Read the model definition and answer for the solid it produces. Units are mm, in the model's axes. Give positions to 0.01 mm unless a question says otherwise; leave off trailing zeros. Loops run counter-clockwise (first coordinate to the right, second up) from the corner with the lowest first, then second, coordinate; pieces in that order, holes last. Notation, with made-up numbers: (87, -36.75) - (141, -36.75) arc R26 cw to (141, -5.75) - close; hole circle Ø5 at (-33.75, 76.25). An arc over 180 degrees is marked (long way). Write each question's results on one line, items separated by ' | '. Start each with the question number.
Q1. The part is cut by section B-B, the plane z = 7. Write down the section's boundary in (x, y) (3 decimals), plus the area to 3 significant figures.
Q2. Given pin 1 (0.8 mm diameter, centred on y = -1, z = 0.5, fed in from -X); pin 2 (1.5 mm diameter, centred on x = 0, y = 0.5, fed in from +Z); pin 3 (1.1 mm diameter, centred on x = -1, z = 0.5, fed in from +Y); pin 4 (0.5 mm diameter, centred on x = 1, z = 0.5, fed in from +Y), each flat-ended and moving along its own axis, determine where each tip first touches the part or whether it passes through.
Q3. Find the intervals of material crossed by line 1 (Y direction, x = -0.25, z = 3); line 2 (Z direction, x = 0, y = -0.1); line 3 (X direction, y = 0.1, z = 0.75), in increasing order. Write a range as from..to.
Q4. The part is cut by section A-A, the plane z = 5. Write down the section's boundary in (x, y).
```python
from build123d import *

# Parameters (mm, degrees)
F0_R     = 2
F1_DEPTH = 1
F2_START = 1
F0_W     = 0.5
F0_H     = 0.5
F2_DEPTH = 0.5
F3_START = 1.5
F3_DEPTH = 8
F4_SIZE2 = 3
F4_SIZE  = 0.75
F6_R     = 0.25


# Not quite as in the source:
# - a fillet or chamfer that OpenCascade refuses, or shapes differently, is made with other operations: its cross-section is extruded or revolved along the edge and cut away or added


with BuildPart() as f1:
    # F0 (on Top) → F1 (new body)
    with BuildSketch(Plane.XY):
        Circle(F0_R)
        with BuildLine():
            ThreePointArc((0.25, 0.9682458366), (0.7071067812, 0.7071067812), (0.9682458366, 0.25))
            Line((0.9682458366, 0.25), (1.25, 0.25))
            Line((1.25, 0.25), (1.25, -0.25))
            Line((1.25, -0.25), (0.9682458366, -0.25))
            ThreePointArc((0.9682458366, -0.25), (0.7071067812, -0.7071067812), (0.25, -0.9682458366))
            Line((0.25, -0.9682458366), (0.25, -1.25))
            Line((0.25, -1.25), (-0.25, -1.25))
            Line((-0.25, -1.25), (-0.25, -0.9682458366))
            ThreePointArc((-0.25, -0.9682458366), (-0.7071067812, -0.7071067812), (-0.9682458366, -0.25))
            Line((-0.9682458366, -0.25), (-1.25, -0.25))
            Line((-1.25, -0.25), (-1.25, 0.25))
            Line((-1.25, 0.25), (-0.9682458366, 0.25))
            ThreePointArc((-0.9682458366, 0.25), (-0.7071067812, 0.7071067812), (-0.25, 0.9682458366))
            Line((-0.25, 0.9682458366), (-0.25, 1.25))
            Line((-0.25, 1.25), (0.25, 1.25))
            Line((0.25, 1.25), (0.25, 0.9682458366))
        make_face(mode=Mode.SUBTRACT)
        with BuildLine():
            Line((-0.25, 0.25), (-0.25, 0.9682458366))
            ThreePointArc((-0.25, 0.9682458366), (-0.7071067812, 0.7071067812), (-0.9682458366, 0.25))
            Line((-0.9682458366, 0.25), (-0.25, 0.25))
        make_face()
        with BuildLine():
            ThreePointArc((-0.9682458366, -0.25), (-0.7071067812, -0.7071067812), (-0.25, -0.9682458366))
            Line((-0.25, -0.9682458366), (-0.25, -0.25))
            Line((-0.25, -0.25), (-0.9682458366, -0.25))
        make_face()
        with BuildLine():
            ThreePointArc((0.25, -0.9682458366), (0.7071067812, -0.7071067812), (0.9682458366, -0.25))
            Line((0.9682458366, -0.25), (0.25, -0.25))
            Line((0.25, -0.25), (0.25, -0.9682458366))
        make_face()
        with BuildLine():
            Line((0.25, 0.25), (0.9682458366, 0.25))
            ThreePointArc((0.9682458366, 0.25), (0.7071067812, 0.7071067812), (0.25, 0.9682458366))
            Line((0.25, 0.9682458366), (0.25, 0.25))
        make_face()
    extrude(amount=F1_DEPTH)

    # F0 (on Top) → F2 (join)
    with BuildSketch(Plane.XY.offset(F2_START)):
        Circle(F0_R)
        with BuildLine():
            ThreePointArc((0.25, 0.9682458366), (0.7071067812, 0.7071067812), (0.9682458366, 0.25))
            Line((0.9682458366, 0.25), (1.25, 0.25))
            Line((1.25, 0.25), (1.25, -0.25))
            Line((1.25, -0.25), (0.9682458366, -0.25))
            ThreePointArc((0.9682458366, -0.25), (0.7071067812, -0.7071067812), (0.25, -0.9682458366))
            Line((0.25, -0.9682458366), (0.25, -1.25))
            Line((0.25, -1.25), (-0.25, -1.25))
            Line((-0.25, -1.25), (-0.25, -0.9682458366))
            ThreePointArc((-0.25, -0.9682458366), (-0.7071067812, -0.7071067812), (-0.9682458366, -0.25))
            Line((-0.9682458366, -0.25), (-1.25, -0.25))
            Line((-1.25, -0.25), (-1.25, 0.25))
            Line((-1.25, 0.25), (-0.9682458366, 0.25))
            ThreePointArc((-0.9682458366, 0.25), (-0.7071067812, 0.7071067812), (-0.25, 0.9682458366))
            Line((-0.25, 0.9682458366), (-0.25, 1.25))
            Line((-0.25, 1.25), (0.25, 1.25))
            Line((0.25, 1.25), (0.25, 0.9682458366))
        make_face(mode=Mode.SUBTRACT)
        with BuildLine():
            Line((0.25, 0.25), (0.25, 0.9682458366))
            ThreePointArc((0.25, 0.9682458366), (0, 1), (-0.25, 0.9682458366))
            Line((-0.25, 0.9682458366), (-0.25, 0.25))
            Line((-0.25, 0.25), (0.25, 0.25))
        make_face()
        with BuildLine():
            ThreePointArc((-0.25, -0.9682458366), (0, -1), (0.25, -0.9682458366))
            Line((0.25, -0.9682458366), (0.25, -0.25))
            Line((0.25, -0.25), (-0.25, -0.25))
            Line((-0.25, -0.25), (-0.25, -0.9682458366))
        make_face()
        with BuildLine():
            ThreePointArc((0.9682458366, -0.25), (0.9920296963, -0.1260042925), (1, 0))
            ThreePointArc((1, 0), (0.9920296963, 0.1260042925), (0.9682458366, 0.25))
            Line((0.9682458366, 0.25), (0.25, 0.25))
            Line((0.25, 0.25), (0.25, -0.25))
            Line((0.25, -0.25), (0.9682458366, -0.25))
        make_face()
        with BuildLine():
            Line((-0.25, -0.25), (-0.25, 0.25))
            Line((-0.25, 0.25), (-0.9682458366, 0.25))
            ThreePointArc((-0.9682458366, 0.25), (-1, 0), (-0.9682458366, -0.25))
            Line((-0.9682458366, -0.25), (-0.25, -0.25))
        make_face()
        with BuildLine():
            ThreePointArc((-0.9682458366, -0.25), (-0.7071067812, -0.7071067812), (-0.25, -0.9682458366))
            Line((-0.25, -0.9682458366), (-0.25, -0.25))
            Line((-0.25, -0.25), (-0.9682458366, -0.25))
        make_face()
        with BuildLine():
            ThreePointArc((0.25, -0.9682458366), (0.7071067812, -0.7071067812), (0.9682458366, -0.25))
            Line((0.9682458366, -0.25), (0.25, -0.25))
            Line((0.25, -0.25), (0.25, -0.9682458366))
        make_face()
        with BuildLine():
            Line((0.25, 0.25), (0.9682458366, 0.25))
            ThreePointArc((0.9682458366, 0.25), (0.7071067812, 0.7071067812), (0.25, 0.9682458366))
            Line((0.25, 0.9682458366), (0.25, 0.25))
        make_face()
        with BuildLine():
            Line((-0.25, 0.25), (-0.25, 0.9682458366))
            ThreePointArc((-0.25, 0.9682458366), (-0.7071067812, 0.7071067812), (-0.9682458366, 0.25))
            Line((-0.9682458366, 0.25), (-0.25, 0.25))
        make_face()
        Rectangle(F0_W, F0_H)
        with BuildLine():
            ThreePointArc((-0.9682458366, -0.25), (-1, 0), (-0.9682458366, 0.25))
            Line((-0.9682458366, 0.25), (-1.25, 0.25))
            Line((-1.25, 0.25), (-1.25, -0.25))
            Line((-1.25, -0.25), (-0.9682458366, -0.25))
        make_face()
        with BuildLine():
            ThreePointArc((0.9682458366, 0.25), (0.9920296963, 0.1260042925), (1, 0))
            ThreePointArc((1, 0), (0.9920296963, -0.1260042925), (0.9682458366, -0.25))
            Line((0.9682458366, -0.25), (1.25, -0.25))
            Line((1.25, -0.25), (1.25, 0.25))
            Line((1.25, 0.25), (0.9682458366, 0.25))
        make_face()
        with BuildLine():
            ThreePointArc((-0.25, 0.9682458366), (0, 1), (0.25, 0.9682458366))
            Line((0.25, 0.9682458366), (0.25, 1.25))
            Line((0.25, 1.25), (-0.25, 1.25))
            Line((-0.25, 1.25), (-0.25, 0.9682458366))
        make_face()
        with BuildLine():
            Line((0.25, -1.25), (0.25, -0.9682458366))
            ThreePointArc((0.25, -0.9682458366), (0, -1), (-0.25, -0.9682458366))
            Line((-0.25, -0.9682458366), (-0.25, -1.25))
            Line((-0.25, -1.25), (0.25, -1.25))
        make_face()
    extrude(amount=F2_DEPTH)

    # F0 (on Top) → F3 (join)
    with BuildSketch(Plane.XY.offset(F3_START)):
        with BuildLine():
            ThreePointArc((-0.9682458366, -0.25), (-0.7071067812, -0.7071067812), (-0.25, -0.9682458366))
            Line((-0.25, -0.9682458366), (-0.25, -0.25))
            Line((-0.25, -0.25), (-0.9682458366, -0.25))
        make_face()
        with BuildLine():
            Line((-0.25, -0.25), (-0.25, 0.25))
            Line((-0.25, 0.25), (-0.9682458366, 0.25))
            ThreePointArc((-0.9682458366, 0.25), (-1, 0), (-0.9682458366, -0.25))
            Line((-0.9682458366, -0.25), (-0.25, -0.25))
        make_face()
        with BuildLine():
            Line((-0.25, 0.25), (-0.25, 0.9682458366))
            ThreePointArc((-0.25, 0.9682458366), (-0.7071067812, 0.7071067812), (-0.9682458366, 0.25))
            Line((-0.9682458366, 0.25), (-0.25, 0.25))
        make_face()
        with BuildLine():
            Line((0.25, 0.25), (0.25, 0.9682458366))
            ThreePointArc((0.25, 0.9682458366), (0, 1), (-0.25, 0.9682458366))
            Line((-0.25, 0.9682458366), (-0.25, 0.25))
            Line((-0.25, 0.25), (0.25, 0.25))
        make_face()
        with BuildLine():
            Line((0.25, 0.25), (0.9682458366, 0.25))
            ThreePointArc((0.9682458366, 0.25), (0.7071067812, 0.7071067812), (0.25, 0.9682458366))
            Line((0.25, 0.9682458366), (0.25, 0.25))
        make_face()
        with BuildLine():
            ThreePointArc((0.9682458366, -0.25), (0.9920296963, -0.1260042925), (1, 0))
            ThreePointArc((1, 0), (0.9920296963, 0.1260042925), (0.9682458366, 0.25))
            Line((0.9682458366, 0.25), (0.25, 0.25))
            Line((0.25, 0.25), (0.25, -0.25))
            Line((0.25, -0.25), (0.9682458366, -0.25))
        make_face()
        with BuildLine():
            ThreePointArc((-0.25, -0.9682458366), (0, -1), (0.25, -0.9682458366))
            Line((0.25, -0.9682458366), (0.25, -0.25))
            Line((0.25, -0.25), (-0.25, -0.25))
            Line((-0.25, -0.25), (-0.25, -0.9682458366))
        make_face()
        with BuildLine():
            ThreePointArc((0.25, -0.9682458366), (0.7071067812, -0.7071067812), (0.9682458366, -0.25))
            Line((0.9682458366, -0.25), (0.25, -0.25))
            Line((0.25, -0.25), (0.25, -0.9682458366))
        make_face()
        Rectangle(F0_W, F0_H)
    extrude(amount=F3_DEPTH)

    # F4
    f4_edges = [f1.edges().sort_by_distance(p)[0] for p in [
        (-0.25, 0.968246, 9.5),
    ]]
    f4_side = f1.faces().sort_by_distance((0, 0, 9.5))[0]
    chamfer(f4_edges, length=F4_SIZE, length2=F4_SIZE2, reference=f4_side)

    # F5: fillet of radius 1 on 1 edges, made by hand

    # F5_s1 → F5_t2 (revolve, cut)
    with BuildSketch(Plane.XZ):
        with BuildLine():
            ThreePointArc((2, 1), (1.7071067812, 0.2928932188), (1, 0))
            Line((1, 0), (2, 0))
            Line((2, 0), (2, 1))
        make_face()
    revolve(axis=Axis((0, 0, 0), (0, 0, 1)), mode=Mode.SUBTRACT)

    # F6
    f6_edges = [f1.edges().sort_by_distance(p)[0] for p in [
        (-2, 0, 1.5),
        (-0.25, 0.968246, 1.5),
    ]]
    fillet(f6_edges, radius=F6_R)


solid = f1.part
```
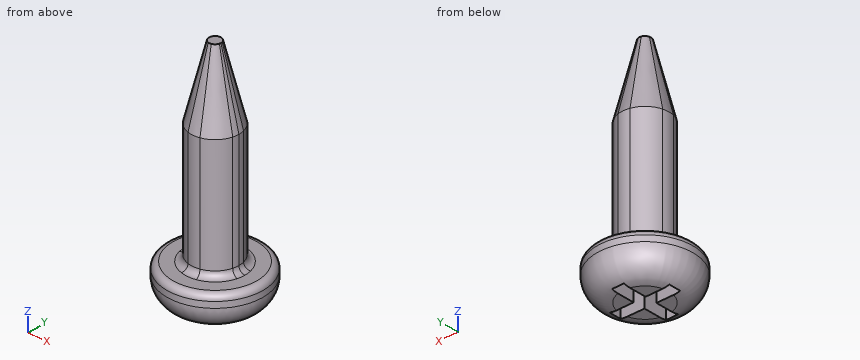
Check sheet entries:
1) outline: circle Ø1.75 at (0, 0) | area: 2.41 mm^2
2) pin 1: stops at x = -1.84 | pin 2: stops at z = 9.5 | pin 3: stops at y = 1.91 | pin 4: stops at y = 1.76
3) line 1: y = -0.97..0.97 | line 2: z = 1..9.5 | line 3: x = -1.97..-1.25, 1.25..1.97
4) outline: circle Ø2 at (0, 0)
